Here's the drawing with two shaded views (mm, measured from the low corner). I have some questions. Coordinates: 2 decimals unless noted, no trailing zeros. Order: outer loops, then holes, each group sorted by start corner. A loop starts at its lowest first (then second) coordinate and runs counter-clockwise, first axis right, second up. Notation, with made-up numbers: (62, 85) -> (112, 85) arc R15 cw to (112, 92) -> close; hole circle Ø10 at (64.5, 67). An arc over 180 degrees is marked (long way). Answer as a JSON object with one key per item and string values. Group by question number.
(1) I want a section at D-D, the plane z = 74. List the corners of the cut face in (x, y) for me.
(2) I want a section at C-C, the plane z = 179. List the corners of the cut face in (x, y) for me (1 decimal).
(3) I want a section at A-A, the plane y = 5. List the corners of the cut face in (x, z) for me.
(4) I need wall thicknesses on line 1 (X direction, y = 11, z = 250); line 2 (Z direction, x = 291.5, y = 15); line 3 (Z direction, x = 195, y = 17) (1 decimal). Which ranges of each line are inside material? Lowest first, please.
(5) I want a section at B-B, the plane x = 250. List the corners of the cut face in (y, z) for me.
(6) For pin 1 (8 mm diameter, centred on x = 361.25, z = 442.69, fed in from +Y); pin 2 (6 mm diameter, centred on x = 192, y = 11, fed in from -Z) (1 decimal); pin 3 (1 mm diameter, centred on x = 98, y = 8.5, fed in from -Z) (1 decimal); pin 4 (2 mm diameter, centred on y = 7, z = 433.5, fed in from -X), each with a flat end and sliding along its axis, tell me the tip position at first contact or that it passes through.
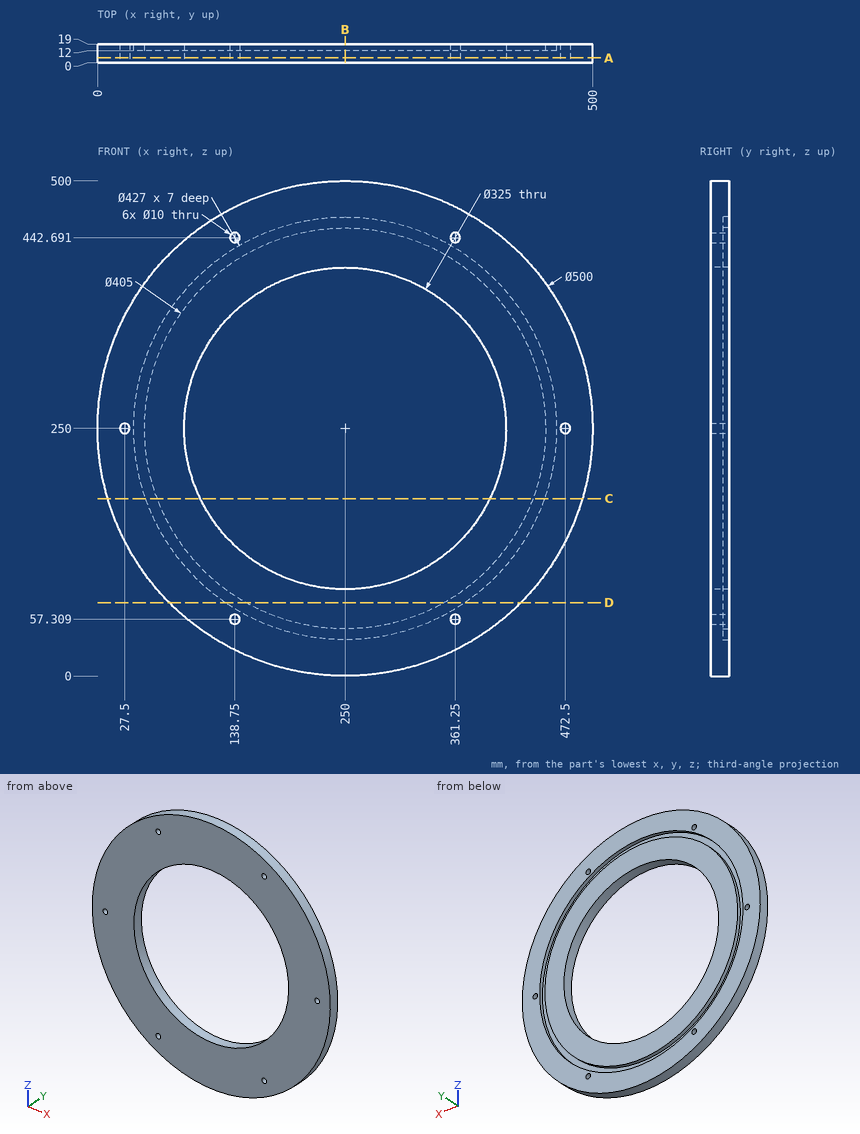
Computed values:
{
 "1": {"outline": "(72.45, 0) -> (427.55, 0) -> (427.55, 19) -> (370.86, 19) -> (370.86, 12) -> (350.15, 12) -> (350.15, 19) -> (149.85, 19) -> (149.85, 12) -> (129.14, 12) -> (129.14, 19) -> (72.45, 19) -> close"},
 "2": {"outline": "(10.3, 0) -> (103.8, 0) -> (103.8, 19) -> (60.4, 19) -> (60.4, 12) -> (48.7, 12) -> (48.7, 19) -> (10.3, 19) -> close; (396.2, 0) -> (489.7, 0) -> (489.7, 19) -> (451.3, 19) -> (451.3, 12) -> (439.6, 12) -> (439.6, 19) -> (396.2, 19) -> close"},
 "3": {"outline": "circle Ø500 at (250, 250); hole circle Ø10 at (27.5, 250); hole circle Ø325 at (250, 250); hole circle Ø10 at (138.75, 57.31); hole circle Ø10 at (138.75, 442.69); hole circle Ø10 at (361.25, 57.31); hole circle Ø10 at (361.25, 442.69); hole circle Ø10 at (472.5, 250)"},
 "4": {"line 1": "x = 0 to 22.5, 32.5 to 87.5, 412.5 to 467.5, 477.5 to 500", "line 2": "z = 3.47 to 40.57, 51.8 to 92.89, 407.11 to 448.2, 459.43 to 496.53", "line 3": "z = 6.1 to 43.7, 55.1 to 97.1, 402.9 to 444.9, 456.3 to 493.9"},
 "5": {"outline": "(0, 0) -> (19, 0) -> (19, 36.5) -> (12, 36.5) -> (12, 47.5) -> (19, 47.5) -> (19, 87.5) -> (0, 87.5) -> close; (0, 412.5) -> (19, 412.5) -> (19, 452.5) -> (12, 452.5) -> (12, 463.5) -> (19, 463.5) -> (19, 500) -> (0, 500) -> close"},
 "6": {"pin 1": "passes through", "pin 2": "stops at z = 6.1", "pin 3": "stops at z = 51.1", "pin 4": "stops at x = 79.14"}
}
